Solid Edge part; units mm, degrees
sketch "Sketch1" plane through (0, 0, 0) normal (0, 0, 1) x (1, 0, 0)
  line L0 (-6.1009, 4.0673) -> (-6.5728, -3.2499)
  line L1 (-6.5728, -3.2499) -> (-0.4719, -7.3171)
  line L2 (-0.4719, -7.3171) -> (6.1009, -4.0673)
  line L3 (6.1009, -4.0673) -> (6.5728, 3.2499)
  line L4 (6.5728, 3.2499) -> (0.4719, 7.3171)
  line L5 (0.4719, 7.3171) -> (-6.1009, 4.0673)
extrude "Protrusion1" add sketch "Sketch1" against normal blind 685
sketch "Sketch2" plane through (0, 0, -2) normal (0, 0, 1) x (-0.8964, -0.4432, 0)
  circle A0 centre (0, 0) radius 5.5
  circle A1 centre (0, 0) radius 13.1424
extrude "ExtrudedCutout_1" cut sketch "Sketch2" against normal blind 2
sketch "Sketch3" plane through (0, 0, -683) normal (0, 0, -1) x (0.8964, 0.4432, 0)
  circle A0 centre (0, 0) radius 5.5
  circle A1 centre (0, 0) radius 13.1424
extrude "ExtrudedCutout_2" cut sketch "Sketch3" against normal blind 2
sketch "Sketch4" plane through (0, 0, -140) normal (0, 0, 1) x (0.8964, 0.4432, 0)
  circle A0 centre (0, 0) radius 5.5
  circle A1 centre (0, 0) radius 13.1424
extrude "ExtrudedCutout_3" cut sketch "Sketch4" along normal blind 2
sketch "Sketch5" plane through (0, 0, -153) normal (0, 0, 1) x (0.8964, 0.4432, 0)
  circle A0 centre (0, 0) radius 5.5
  circle A1 centre (0, 0) radius 10.4372
extrude "ExtrudedCutout_4" cut sketch "Sketch5" against normal blind 2
properties part number "BumbleB0932"
Verification items for the finished model (mm, model axes). Give positions to 0.01 mm unless a question says otherwise; leave off trailing zeros. Order: outer loops, then holes, each group sorted by start corner. A loop starts at its lowest first (then second) coordinate and runs counter-clockwise, first axis right, second up. Notation, with made-up numbers: (23, 7) - (72, 7) arc R21 ccw to (72, 46) - close; hole circle Ø8 at (42.5, -32.75). An arc over 180 degrees is marked (long way). Answer as CSV lines item,"result". Start each with the question number.
Item 1: Section check A-A, the plane z = -89. Record the boundary of the cut face in (x, y).
Item 2: Material ranges on L1, parallel to Z at x = 4.75, y = 3.75; L2, parallel to X at y = 2.5, z = -520; L3, parallel to Y at x = -2.25, z = -134, recorded low to high.
Item 3: Mould release check, pull along Z, two halves, no side actions. Record for faces 1 (the face through (5.49, 0.36, -153.99)), 2 (the face through (0, 0, -685)), 3 (the face through (0, 0, 0)): released by +Z, released by -Z, zero draft, split by the parting line, or undercut.
Item 4: Gauge pin test, flat ends, axial feed: pin 1 (4 mm diameter, centred on x = 1, y = 2, fed in from +Z); pin 2 (4 mm diameter, centred on y = -5.5, z = -496.5, fed in from -X); pin 3 (1.5 mm diameter, centred on x = -4, z = -417, fed in from -Y); pin 4 (1 mm diameter, centred on y = 1, z = -613.5, fed in from +X). Record the tip position at first contact, or that the pin passes through.
Filled in:
1,outline,"(-6.57, -3.25) - (-0.47, -7.32) - (6.1, -4.07) - (6.57, 3.25) - (0.47, 7.32) - (-6.1, 4.07) - close"
2,L1,"-685 to -683, -681 to -155, -153 to -140, -138 to -4, -2 to 0"
2,L2,"-6.2 to 6.52"
2,L3,"-6.13 to 5.97"
3,face 1,"undercut"
3,face 2,"released by -Z"
3,face 3,"released by +Z"
4,pin 1,"z = 0"
4,pin 2,"x = -6.2"
4,pin 3,"y = -5.47"
4,pin 4,"x = 6.46"
